```python
from build123d import *

# Parameters (mm, degrees)
F0_R     = 19.6
F0_R_2   = 8.025
F1_DEPTH = 5
F3_DEPTH = 8.5
F4_DEPTH = 5.001


with BuildPart() as f1:
    # F0 (on Top) → F1 (new body)
    with BuildSketch(Plane.XY):
        Circle(F0_R)
        Circle(F0_R_2, mode=Mode.SUBTRACT)
    extrude(amount=F1_DEPTH)

    # F2 (on face) → F3 (join)
    with BuildSketch(Plane.XY.offset(5)):
        with BuildLine():
            ThreePointArc((-13.2966161109, -14.4), (0, -19.6), (13.2966161109, -14.4))
            Line((13.2966161109, -14.4), (-13.2966161109, -14.4))
        make_face()
        with BuildLine():
            Line((-13.2966161109, 14.4), (13.2966161109, 14.4))
            ThreePointArc((13.2966161109, 14.4), (0, 19.6), (-13.2966161109, 14.4))
        make_face()
    extrude(amount=F3_DEPTH)

    # F2 (on face) → F4 (cut, through all)
    with BuildSketch(Plane.XY.offset(5)):
        with BuildLine():
            ThreePointArc((-14.4, 13.2966161109), (-19.6, 0), (-14.4, -13.2966161109))
            Line((-14.4, -13.2966161109), (-14.4, 13.2966161109))
        make_face()
        with BuildLine():
            Line((14.4, 13.2966161109), (14.4, -13.2966161109))
            ThreePointArc((14.4, -13.2966161109), (18.2537667346, -7.138627319), (19.6, 0))
            ThreePointArc((19.6, 0), (18.2537667346, 7.138627319), (14.4, 13.2966161109))
        make_face()
    extrude(amount=-F4_DEPTH, mode=Mode.SUBTRACT)


solid = f1.part
```
Build history of the part. All positions in model axes, mm. A direction names the side the tool comes from. Round coordinates to 2 decimals unless told otherwise and drop trailing zeros. Write each loop counter-clockwise with the first axis right and the second up, starting at its lowest first coordinate (ties: lowest second). Pieces come first, ordered by that corner, then holes.
1) Band-saw the part on D-D, the plane z = 3.25. List the corners of the cut face in (x, y) (3 decimals), and give its area (3 significant figures).
2) Band-saw the part on A-A, the plane y = 0. List the corners of the cut face in (x, z) (3 decimals).
3) Pin check, flat tips, straight feed: pin 1 (12 mm diameter, centred on x = -6.5, y = 2, fed in from +Z); pin 2 (13 mm diameter, centred on x = 0, y = 0, fed in from -Z); pin 3 (7 mm diameter, centred on x = 5.5, z = 7, fed in from +Y). Stop position of each tip, or through.
4) 3-axis set-ups, long thin cutter, end or side, ignore diameter. For faces 5 (the flat face through (0, 14.4, 9)), 6 (the flat face through (0, -16, 13.5)): which of +Z, -Z, +X, -X, +Y, -Y reach the whole face in a straight line?
5) Band-saw the part on C-C, the plane z = 9.75. List the corners of the cut face in (x, y).
6) Drill centre lines: probe 1 along Y at (x, z) = (0.5, 11.25); probe 2 along Z at (x, y) = (-8.75, 0); probe 3 along Y at (x, z) = (5.5, 10). Where is each one in solid material? Low to high.
7) Mould opens along X. For faces 1 (the flat face through (-7, -6, 5)), 2 (the flat face through (-14.4, 0, 3)), 3 (the cylindrical face through (-6.37, -4.88, 2.46)), 4 (the flat face through (14.4, 0, 3)) say: +X half, -X half, draft (parallel to the pull), parting line (faces both ways), or undercut.
8) Band-saw the part on B-B, the plane x = 0. List the corners of the cut face in (y, z) (3 decimals), and give its area (3 significant figures).
Ans:
1. outline: (-14.4, -13.297) arc R19.6 ccw to (14.4, -13.297) - (14.4, 13.297) arc R19.6 ccw to (-14.4, 13.297) - close; hole circle Ø16.05 at (0, 0)
1. area: 815 mm2
2. outline: (-14.4, 0) - (-8.025, 0) - (-8.025, 5) - (-14.4, 5) - close; (8.025, 0) - (14.4, 0) - (14.4, 5) - (8.025, 5) - close
3. pin 1: stops at z = 5
3. pin 2: passes through
3. pin 3: stops at y = 19.5
4. face 5: +Z, +X, -X
4. face 6: +Z, +X, -X, +Y, -Y
5. outline: (-13.3, -14.4) arc R19.6 ccw to (13.3, -14.4) - close; (-13.3, 14.4) - (13.3, 14.4) arc R19.6 ccw to start
6. probe 1: y = -19.59 to -14.4, 14.4 to 19.59
6. probe 2: z = 0 to 5
6. probe 3: y = -18.81 to -14.4, 14.4 to 18.81
7. face 1: draft
7. face 2: -X half
7. face 3: undercut
7. face 4: +X half
8. outline: (-19.6, 0) - (-8.025, 0) - (-8.025, 5) - (-14.4, 5) - (-14.4, 13.5) - (-19.6, 13.5) - close; (8.025, 0) - (19.6, 0) - (19.6, 13.5) - (14.4, 13.5) - (14.4, 5) - (8.025, 5) - close
8. area: 204 mm2
